Verification items for the finished model (mm, model axes). Face numbers are marked on the shaded views. A direction names the side the tool comes from. Coordinates: 2 decimals unless noted, no trailing zeros. Use CSV: the item, a comma, the result in double quotes. Start each with the question number.
1) Tool access check on the marked faces 1 and 2. Record the directions out of +Z, -Z, +X, -X, +Y, -Y that give a thin tool (end or side, any length) a straight path to the whole face; none if there is none.
2) Release check for a two-part mould opening along Z. For the marked faces 3 and 4 record: released by +Z, released by -Z, zero draft, split by the parting line, or undercut.
3) Scan lines: line 1 along X through (y, z) = (-1.2, 0); line 2 along X through (y, z) = (-1.15, -13); line 3 along X through (y, z) = (-4.45, 0). Record each from-to range of solid material in increasing order.
4) Go/stop test with flat-tipped pins: pin 1 (4.5 mm diameter, centred on x = 19, z = 0, fed in from +Y); pin 2 (6 mm diameter, centred on x = 0, z = -19, fed in from +Y); pin 3 (2 mm diameter, centred on x = 10.5, y = -3, fed in from +Z); pin 4 (1 mm diameter, centred on y = -1, z = 7, fed in from -X). Record where each tip stops, or that it passes through.
5) Sectioned sample at A-A on x = 0. Give the number of separate pieces and of enclosed holes in the cut face, then the cut area to 3 significant figures.
from build123d import *

# Parameters (mm, degrees)
SKETCH2_R           = 23.75
SKETCH2_R_2         = 2.5
SKETCH2_R_3         = 1.5875
BOSS_EXTRUDE2_DEPTH = 5
SKETCH3_R           = 3.45
CUT_EXTRUDE1_DEPTH  = 4
SKETCH5_R           = 2
CUT_EXTRUDE2_DEPTH  = 10
SKETCH6_R           = 4
CUT_EXTRUDE3_DEPTH  = 4
CHAMFER2_SIZE       = 1
SKETCH7_R           = 24.75
SKETCH7_R_2         = 2.5
SKETCH7_R_3         = 1.5875
SKETCH7_R_4         = 3.45
BOSS_EXTRUDE3_DEPTH = 0.25
CHAMFER3_SIZE       = 0.5
CIRPATTERN1_COUNT   = 12


with BuildPart() as part:
    # Sketch2 → Boss-Extrude2 (new body)
    with BuildSketch(Plane(origin=(0, 0, 0), x_dir=(-1, 0, 0), z_dir=(0, 1, 0))):
        with Locations(Location((0, 0, 0), (0, 0, 90))):
            Circle(SKETCH2_R)
        with Locations(Location((-13.435028843, 13.435028843, 0), (0, 0, 90))):
            Circle(SKETCH2_R_2, mode=Mode.SUBTRACT)
        with Locations(Location((13.435028843, 13.435028843, 0), (0, 0, 90))):
            Circle(SKETCH2_R_2, mode=Mode.SUBTRACT)
        with Locations(Location((0, 0, 0), (0, 0, 90))):
            Circle(SKETCH2_R_3, mode=Mode.SUBTRACT)
        with Locations(Location((13.435028843, -13.435028843, 0), (0, 0, 90))):
            Circle(SKETCH2_R_2, mode=Mode.SUBTRACT)
        with Locations(Location((0, 19, 0), (0, 0, 90))):
            Circle(SKETCH2_R_2, mode=Mode.SUBTRACT)
        with Locations(Location((19, 0, 0), (0, 0, 90))):
            Circle(SKETCH2_R_2, mode=Mode.SUBTRACT)
        with Locations(Location((0, -19, 0), (0, 0, 90))):
            Circle(SKETCH2_R_2, mode=Mode.SUBTRACT)
        with Locations(Location((-19, 0, 0), (0, 0, 90))):
            Circle(SKETCH2_R_2, mode=Mode.SUBTRACT)
        with Locations(Location((-13.435028843, -13.435028843, 0), (0, 0, 90))):
            Circle(SKETCH2_R_2, mode=Mode.SUBTRACT)
    extrude(amount=-BOSS_EXTRUDE2_DEPTH)

    # Sketch3 → Cut-Extrude1 (cut)
    with BuildSketch(Plane(origin=(0, 0, 0), x_dir=(1, 0, 0), z_dir=(0, 1, 0))):
        with Locations(Location((0, 19, 0), (0, 0, 270))):
            Circle(SKETCH3_R)
        with Locations(Location((19, 0, 0), (0, 0, 270))):
            Circle(SKETCH3_R)
        with Locations(Location((0, -19, 0), (0, 0, 270))):
            Circle(SKETCH3_R)
        with Locations(Location((-19, 0, 0), (0, 0, 270))):
            Circle(SKETCH3_R)
    extrude(amount=-CUT_EXTRUDE1_DEPTH, mode=Mode.SUBTRACT)

    # Sketch4 → Revolve1 (revolve)
    with BuildSketch(Plane.XY, mode=Mode.PRIVATE) as revolve1_sk:
        with BuildLine():
            Line((-24.75, 0), (-23.75, 0))
            Line((-23.75, 0), (-23.75, -5))
            Line((-23.75, -5), (-24.75, -5))
            Line((-24.75, -5), (-24.75, -3.618033989))
            ThreePointArc((-24.75, -3.618033989), (-24.25, -2.5), (-24.75, -1.381966011))
            Line((-24.75, -1.381966011), (-24.75, 0))
        make_face()
        with BuildLine():
            Line((-26.75, -5), (-26.75, -3.618033989))
            ThreePointArc((-26.75, -3.618033989), (-27.25, -2.5), (-26.75, -1.381966011))
            Line((-26.75, -1.381966011), (-26.75, 0))
            Line((-26.75, 0), (-35, 0))
            Line((-35, 0), (-35, -5))
            Line((-35, -5), (-26.75, -5))
        make_face()
    revolve(revolve1_sk.sketch.rotate(Axis((0, -2.5, 0), (0, 1, 0)), 270), axis=Axis((0, -2.5, 0), (0, 1, 0)))


with BuildPart() as revolve1_piece_1:
    # of the separate pieces the step leaves, piece 1, a body of its own (revolve1_pieces)
    add(part.part.solids().sort_by_distance((13.435028843, 0, -10.935028843))[0])

    # Sketch7 → Boss-Extrude3 (add)
    with BuildSketch(Plane(origin=(0, 0, 0), x_dir=(1, 0, 0), z_dir=(0, 1, 0))):
        with Locations(Location((0, 0, 0), (0, 0, 90))):
            Circle(SKETCH7_R)
        with Locations(Location((13.435028843, 13.435028843, 0), (0, 0, 270))):
            Circle(SKETCH7_R_2, mode=Mode.SUBTRACT)
        with Locations(Location((-13.435028843, 13.435028843, 0), (0, 0, 270))):
            Circle(SKETCH7_R_2, mode=Mode.SUBTRACT)
        with Locations(Location((0, 0, 0), (0, 0, 270))):
            Circle(SKETCH7_R_3, mode=Mode.SUBTRACT)
        with Locations(Location((-13.435028843, -13.435028843, 0), (0, 0, 270))):
            Circle(SKETCH7_R_2, mode=Mode.SUBTRACT)
        with Locations(Location((13.435028843, -13.435028843, 0), (0, 0, 270))):
            Circle(SKETCH7_R_2, mode=Mode.SUBTRACT)
        with Locations(Location((-19, 0, 0), (0, 0, 270))):
            Circle(SKETCH7_R_4, mode=Mode.SUBTRACT)
        with Locations(Location((0, -19, 0), (0, 0, 270))):
            Circle(SKETCH7_R_4, mode=Mode.SUBTRACT)
        with Locations(Location((19, 0, 0), (0, 0, 270))):
            Circle(SKETCH7_R_4, mode=Mode.SUBTRACT)
        with Locations(Location((0, 19, 0), (0, 0, 270))):
            Circle(SKETCH7_R_4, mode=Mode.SUBTRACT)
    extrude(amount=BOSS_EXTRUDE3_DEPTH)

    # Chamfer3
    chamfer3_edges = [revolve1_piece_1.edges().sort_by_distance(p)[0] for p in [
        (0, 0.25, 24.75),
        (13.435028843, 0.25, -15.935028843),
        (-13.435028843, 0.25, -15.935028843),
        (0, 0.25, -1.5875),
        (-13.435028843, 0.25, 10.935028843),
        (13.435028843, 0.25, 10.935028843),
        (-19, 0.25, -3.45),
        (0, 0.25, 15.55),
        (19, 0.25, -3.45),
        (0, 0.25, -22.45),
    ]]
    chamfer(chamfer3_edges, length=CHAMFER3_SIZE)


with BuildPart() as revolve1_piece_2:
    # of the separate pieces the step leaves, piece 2, a body of its own (revolve1_pieces)
    add(part.part.solids().sort_by_distance((0, -5, -26.75))[0])

    # Sketch5 → Cut-Extrude2 (cut)
    with BuildSketch(Plane(origin=(0, 0, 0), x_dir=(1, 0, 0), z_dir=(0, 1, 0))):
        with Locations(Location((0, 32.5, 0), (0, 0, 270))):
            Circle(SKETCH5_R)
        with Locations(Location((32.5, 0, 0), (0, 0, 270))):
            Circle(SKETCH5_R)
        with Locations(Location((0, -32.5, 0), (0, 0, 270))):
            Circle(SKETCH5_R)
        with Locations(Location((-32.5, 0, 0), (0, 0, 270))):
            Circle(SKETCH5_R)
    extrude(amount=-CUT_EXTRUDE2_DEPTH, mode=Mode.SUBTRACT)

    # Sketch6 → Cut-Extrude3 (cut)
    with BuildSketch(Plane(origin=(0, 0, 0), x_dir=(1, 0, 0), z_dir=(0, 1, 0))):
        with Locations((0, -32.5)):
            Circle(SKETCH6_R)
        with Locations((-32.5, 0)):
            Circle(SKETCH6_R)
        with Locations((0, 32.5)):
            Circle(SKETCH6_R)
        with Locations((32.5, 0)):
            Circle(SKETCH6_R)
    extrude(amount=-CUT_EXTRUDE3_DEPTH, mode=Mode.SUBTRACT)

    # Chamfer2
    # the kernel refuses this chamfer: 1 mm, written as the material it takes off along each edge
    with BuildSketch(Plane(origin=(0, 0, 0), x_dir=(0.019114321981189532, 0, 0.9998173046588058), z_dir=(-0.9998173046588058, 0, 0.019114321981189532))) as chamfer2_piece_1:
        Polygon((35 - CHAMFER2_SIZE, 0), (35, -CHAMFER2_SIZE), (35, 0), align=None)
    revolve(axis=Axis((0, 0, 0), (0, 1, 0)), revolution_arc=87.809526646, mode=Mode.SUBTRACT)
    with BuildSketch(Plane(origin=(0, 0, 0), x_dir=(-0.9998173046588067, 0, 0.019114321981147413), z_dir=(-0.019114321981147413, 0, -0.9998173046588067))) as chamfer2_piece_2:
        Polygon((35 - CHAMFER2_SIZE, 0), (35, -CHAMFER2_SIZE), (35, 0), align=None)
    revolve(axis=Axis((0, 0, 0), (0, 1, 0)), revolution_arc=87.809526646, mode=Mode.SUBTRACT)
    with BuildSketch(Plane(origin=(0, 0, 0), x_dir=(-0.019114321981182705, 0, -0.999817304658806), z_dir=(0.999817304658806, 0, -0.019114321981182705))) as chamfer2_piece_3:
        Polygon((35 - CHAMFER2_SIZE, 0), (35, -CHAMFER2_SIZE), (35, 0), align=None)
    revolve(axis=Axis((0, 0, 0), (0, 1, 0)), revolution_arc=87.809526646, mode=Mode.SUBTRACT)
    with BuildSketch(Plane(origin=(0, 0, 32.5), x_dir=(-0.29349569960602556, -1.3653955404004917e-15, 0.9559603936946184), z_dir=(0.9559603936946184, 1.4794691735989965e-15, 0.29349569960602556))) as chamfer2_piece_4:
        Polygon((4 + CHAMFER2_SIZE, 0), (4, CHAMFER2_SIZE), (4, 0), align=None)
    revolve(axis=Axis((0, 0, 32.5), (0, -1, 0)), revolution_arc=325.865290322, mode=Mode.SUBTRACT)
    with BuildSketch(Plane(origin=(-32.5, 0, 0), x_dir=(-0.9559603936947099, -1.386827160904714e-15, -0.2934956996057275), z_dir=(-0.2934956996057275, 7.472387430751279e-15, 0.9559603936947099))) as chamfer2_piece_5:
        Polygon((4 + CHAMFER2_SIZE, 0), (4, CHAMFER2_SIZE), (4, 0), align=None)
    revolve(axis=Axis((-32.5, 0, 0), (0, -1, 0)), revolution_arc=325.865290322, mode=Mode.SUBTRACT)
    with BuildSketch(Plane(origin=(0, 0, 0), x_dir=(0.9998173046588067, 0, -0.0191143219811504), z_dir=(0.0191143219811504, 0, 0.9998173046588067))) as chamfer2_piece_6:
        Polygon((35 - CHAMFER2_SIZE, 0), (35, -CHAMFER2_SIZE), (35, 0), align=None)
    revolve(axis=Axis((0, 0, 0), (0, 1, 0)), revolution_arc=87.809526646, mode=Mode.SUBTRACT)
    with BuildSketch(Plane(origin=(0, 0, -32.5), x_dir=(-0.29349569960600574, -1.3653955404004456e-15, -0.9559603936946244), z_dir=(0.9559603936946244, 1.4794691735989516e-15, -0.29349569960600574))) as chamfer2_piece_7:
        Polygon((4 + CHAMFER2_SIZE, 0), (4, -CHAMFER2_SIZE), (4, 0), align=None)
    revolve(axis=Axis((0, 0, -32.5), (0, 1, 0)), revolution_arc=325.865290322, mode=Mode.SUBTRACT)
    with BuildSketch(Plane(origin=(0, 0, 0), x_dir=(0, 0, -1), z_dir=(1, 0, 0))) as chamfer2_piece_8:
        Polygon((26.75, -CHAMFER2_SIZE), (26.75 + CHAMFER2_SIZE, 0), (26.75, 0), align=None)
    revolve(axis=Axis((0, 0, 0), (0, 1, 0)), mode=Mode.SUBTRACT)
    with BuildSketch(Plane(origin=(32.5, 0, 0), x_dir=(0.9559603936946928, 0, -0.2934956996057833), z_dir=(0.2934956996057833, 0, 0.9559603936946928))) as chamfer2_piece_9:
        Polygon((4 + CHAMFER2_SIZE, 0), (4, -CHAMFER2_SIZE), (4, 0), align=None)
    revolve(axis=Axis((32.5, 0, 0), (0, 1, 0)), revolution_arc=325.865290322, mode=Mode.SUBTRACT)


with BuildPart() as body_3:
    # Sketch8 → Revolve2 (revolve)
    with BuildSketch(Plane.XY):
        with BuildLine():
            Line((25.75, -1), (25.75, -4))
            ThreePointArc((25.75, -4), (24.25, -2.5), (25.75, -1))
        make_face()
    revolve(axis=Axis((25.75, -1, 0), (0, -1, 0)))


with BuildPart() as cirpattern1_1:
    # CirPattern1: pattern copy
    add(body_3.part.rotate(Axis((0, 0, 0), (0, 1, 0)), 1 * 360 / CIRPATTERN1_COUNT))


with BuildPart() as cirpattern1_2:
    # CirPattern1: pattern copy
    add(body_3.part.rotate(Axis((0, 0, 0), (0, 1, 0)), 2 * 360 / CIRPATTERN1_COUNT))


with BuildPart() as cirpattern1_3:
    # CirPattern1: pattern copy
    add(body_3.part.rotate(Axis((0, 0, 0), (0, 1, 0)), 3 * 360 / CIRPATTERN1_COUNT))


with BuildPart() as cirpattern1_4:
    # CirPattern1: pattern copy
    add(body_3.part.rotate(Axis((0, 0, 0), (0, 1, 0)), 4 * 360 / CIRPATTERN1_COUNT))


with BuildPart() as cirpattern1_5:
    # CirPattern1: pattern copy
    add(body_3.part.rotate(Axis((0, 0, 0), (0, 1, 0)), 5 * 360 / CIRPATTERN1_COUNT))


with BuildPart() as cirpattern1_6:
    # CirPattern1: pattern copy
    add(body_3.part.rotate(Axis((0, 0, 0), (0, 1, 0)), 6 * 360 / CIRPATTERN1_COUNT))


with BuildPart() as cirpattern1_7:
    # CirPattern1: pattern copy
    add(body_3.part.rotate(Axis((0, 0, 0), (0, 1, 0)), 7 * 360 / CIRPATTERN1_COUNT))


with BuildPart() as cirpattern1_8:
    # CirPattern1: pattern copy
    add(body_3.part.rotate(Axis((0, 0, 0), (0, 1, 0)), 8 * 360 / CIRPATTERN1_COUNT))


with BuildPart() as cirpattern1_9:
    # CirPattern1: pattern copy
    add(body_3.part.rotate(Axis((0, 0, 0), (0, 1, 0)), 9 * 360 / CIRPATTERN1_COUNT))


with BuildPart() as cirpattern1_10:
    # CirPattern1: pattern copy
    add(body_3.part.rotate(Axis((0, 0, 0), (0, 1, 0)), 10 * 360 / CIRPATTERN1_COUNT))


with BuildPart() as cirpattern1_11:
    # CirPattern1: pattern copy
    add(body_3.part.rotate(Axis((0, 0, 0), (0, 1, 0)), 11 * 360 / CIRPATTERN1_COUNT))


solid = revolve1_piece_1.part
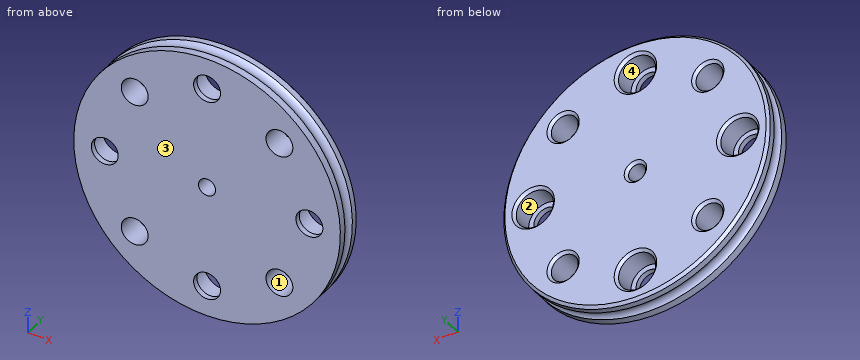
Answers follow:
1,face 1,"+Y, -Y"
1,face 2,"+Y"
2,face 3,"zero draft"
2,face 4,"undercut"
3,line 1,"x = -24.75 to -22.45, -15.55 to -1.59, 1.59 to 15.55, 22.45 to 24.75"
3,line 2,"x = -21.06 to -15.9, -10.97 to 10.97, 15.9 to 21.06"
3,line 3,"x = -24.75 to -21.5, -16.5 to -1.59, 1.59 to 16.5, 21.5 to 24.75"
4,pin 1,"passes through"
4,pin 2,"stops at y = -4"
4,pin 3,"stops at z = 22.76"
4,pin 4,"stops at x = -23.88"
5,separate pieces,"4"
5,enclosed holes,"0"
5,area,"172 mm²"
